Input: part model. Units: mm. Frame: model coordinates. Face numbers are marked on the shaded views. Round coordinates to 2 decimals unless told otherwise and drop trailing zeros. Order: outer loops, then holes, each group sorted by start corner. A loop starts at its lowest first (then second) coordinate and runs counter-clockwise, first axis right, second up.
Item 1: Cut plane D-D on z = -51.5. Output: boundary loops of the cut face in (x, y).
Item 2: Cut plane C-C on x = 12. Output: boundary loops of the cut face in (y, z), then the cut area to 3 significant figures.
Item 3: Cut plane B-B on z = -20. Output: boundary loops of the cut face in (x, y), then the cut area to 3 significant figures.
Item 4: Cut plane A-A on y = 11. Output: boundary loops of the cut face in (x, z).
Item 5: First-contact query: pin 1 (10 mm diameter, centred on x = 30.5, z = -45, fed in from -Y). Flat tip, straight axial feed; report the tip coordinate or a pass-through.
Item 6: Mould query, pull axis X, two halves, no side actions, for the marked faces 1, 2, 3 and 4. Classes: released by +X, released by -X, zero draft, split by the parting line, or undercut.
Item 7: Line query: L1, parallel to X at y = 20.3, z = -163; L2, parallel to X at y = 20.2, z = -7.5; L3, parallel to X at y = 13.5, z = -129. Output: solid intervals per line, ascending.
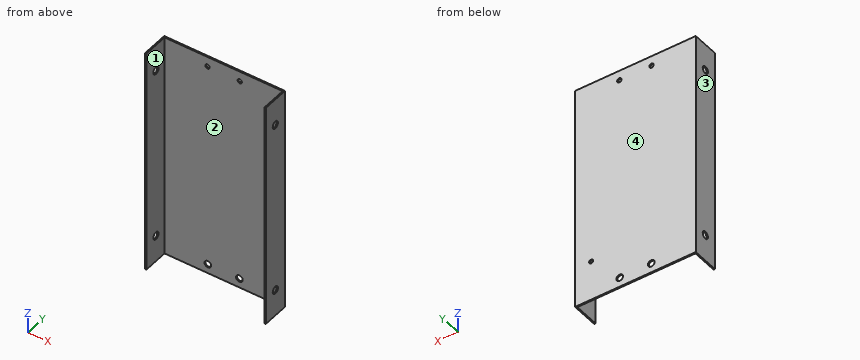
```python
from build123d import *

# Parameters (mm, degrees)
BOSS_EXTRUDE1_DEPTH = 170
SKETCH2_R           = 2.75
CUT_EXTRUDE1_DEPTH  = 90
SKETCH3_R           = 1.65
CUT_EXTRUDE2_DEPTH  = 10
CUT_EXTRUDE3_REACH  = 178.989
SKETCH4_R           = 2.5
CUT_EXTRUDE4_REACH  = 178.989
SKETCH5_R           = 1.5


with BuildPart() as part:
    # Sketch1 → Boss-Extrude1 (new body)
    with BuildSketch(Plane.XY):
        Polygon((-45, 1), (-45, 21), (45, 21), (45, 1), (44, 1), (44, 20), (-44, 20), (-44, 1), align=None)
    extrude(amount=-BOSS_EXTRUDE1_DEPTH)

    # Sketch2 → Cut-Extrude1 (cut)
    with BuildSketch(Plane.ZY.offset(45)):
        with Locations((-150, 11)):
            Circle(SKETCH2_R)
        with Locations((-20, 11)):
            Circle(SKETCH2_R)
    extrude(amount=-CUT_EXTRUDE1_DEPTH, mode=Mode.SUBTRACT)

    # Sketch3 → Cut-Extrude2 (cut)
    with BuildSketch(Plane(origin=(0, 21, 0), x_dir=(1, 0, 0), z_dir=(0, 1, 0))):
        with Locations(Location((12, 7.5, 0), (0, 0, 270))):
            Circle(SKETCH3_R)
        with Locations((-12, 7.5)):
            Circle(SKETCH3_R)
    extrude(amount=-CUT_EXTRUDE2_DEPTH, mode=Mode.SUBTRACT)

    # Sketch4 → Cut-Extrude3 (cut, up to next)
    with BuildSketch(Plane(origin=(0, 21, 0), x_dir=(1, 0, 0), z_dir=(0, 1, 0)), mode=Mode.PRIVATE) as cut_extrude3_sk1:
        with Locations(Location((-11.75, 163, 0), (0, 0, 270))):
            Circle(SKETCH4_R)
    cut_extrude3_tool1 = extrude(cut_extrude3_sk1.sketch, amount=-CUT_EXTRUDE3_REACH, mode=Mode.PRIVATE) & part.part
    # Sketch4 → Cut-Extrude3 (cut, up to next)
    with BuildSketch(Plane(origin=(0, 21, 0), x_dir=(1, 0, 0), z_dir=(0, 1, 0)), mode=Mode.PRIVATE) as cut_extrude3_sk2:
        with Locations((11.75, 163)):
            Circle(SKETCH4_R)
    cut_extrude3_tool2 = extrude(cut_extrude3_sk2.sketch, amount=-CUT_EXTRUDE3_REACH, mode=Mode.PRIVATE) & part.part
    add(cut_extrude3_tool1.solids().sort_by_distance((-11.75, 21, -163))[0], mode=Mode.SUBTRACT)
    add(cut_extrude3_tool2.solids().sort_by_distance((11.75, 21, -163))[0], mode=Mode.SUBTRACT)

    # Sketch5 → Cut-Extrude4 (cut, up to next)
    with BuildSketch(Plane(origin=(0, 21, 0), x_dir=(1, 0, 0), z_dir=(0, 1, 0)), mode=Mode.PRIVATE) as cut_extrude4_sk1:
        with Locations(Location((33, 140, 0), (0, 0, 270))):
            Circle(SKETCH5_R)
    cut_extrude4_tool1 = extrude(cut_extrude4_sk1.sketch, amount=-CUT_EXTRUDE4_REACH, mode=Mode.PRIVATE) & part.part
    add(cut_extrude4_tool1.solids().sort_by_distance((33, 21, -140))[0], mode=Mode.SUBTRACT)


solid = part.part
```
From the geometry:
1. outline: (-45, 1) - (-44, 1) - (-44, 20) - (44, 20) - (44, 1) - (45, 1) - (45, 21) - (-45, 21) - close
2. outline: (20, -170) - (21, -170) - (21, -165.49) - (20, -165.49) - close; (20, -160.51) - (21, -160.51) - (21, -9.15) - (20, -9.15) - close; (20, -5.85) - (21, -5.85) - (21, 0) - (20, 0) - close
2. area: 162 mm2
3. outline: (-45, 1) - (-44, 1) - (-44, 8.25) - (-45, 8.25) - close; (-45, 13.75) - (-44, 13.75) - (-44, 20) - (44, 20) - (44, 13.75) - (45, 13.75) - (45, 21) - (-45, 21) - close; (44, 1) - (45, 1) - (45, 8.25) - (44, 8.25) - close
3. area: 117 mm2
4. outline: (-45, -170) - (-44, -170) - (-44, -152.75) - (-45, -152.75) - close; (-45, -147.25) - (-44, -147.25) - (-44, -22.75) - (-45, -22.75) - close; (-45, -17.25) - (-44, -17.25) - (-44, 0) - (-45, 0) - close; (44, -170) - (45, -170) - (45, -152.75) - (44, -152.75) - close; (44, -147.25) - (45, -147.25) - (45, -22.75) - (44, -22.75) - close; (44, -17.25) - (45, -17.25) - (45, 0) - (44, 0) - close
5. pin 1: stops at y = 20
6. face 1: undercut
6. face 2: undercut
6. face 3: released by -X
6. face 4: zero draft
7. L1: x = -45 to -14.25, -9.25 to 9.25, 14.25 to 45
7. L2: x = -45 to -13.65, -10.35 to 10.35, 13.65 to 45
7. L3: x = -45 to -44, 44 to 45
